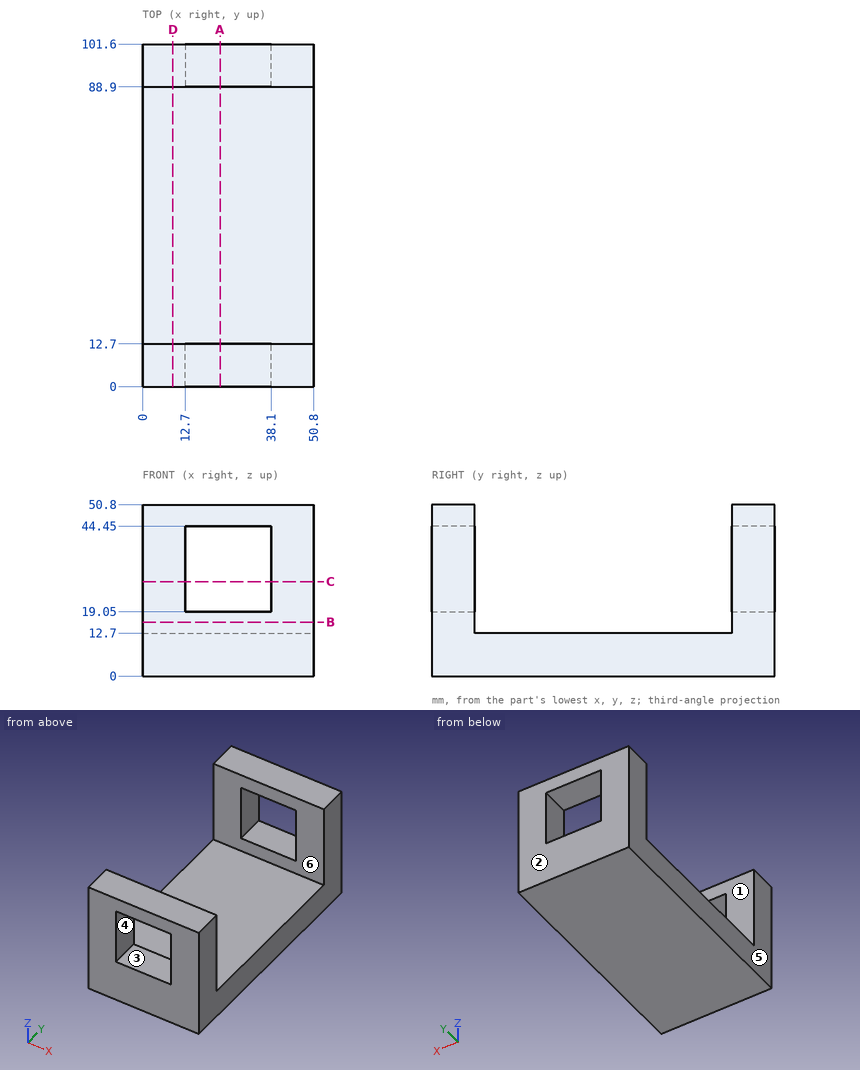
Design review of the part shown in the three views and the two pictorial views. Dimensions are in mm from the part's minimum x, y and z. A direction names the side the tool comes from. Give positions to 0.01 mm unless a question says otherwise; leave off trailing zeros. Loops run counter-clockwise (first coordinate to the right, second up) from the corner with the lowest first, then second, coordinate; pieces in that order, holes last. Notation, with made-up numbers: (-4.5, -3.5) -> (10.5, -3.5) arc R37 ccw to (10.5, 34.5) -> close; hole circle Ø3 at (54, 20). An arc over 180 degrees is marked (long way). Put each result on its own line as item: value. Start each with the question number.
1. Mouldability with a two-part tool opening along Y and no side actions: class the marked faces 1, 2 and 3 as released by +Y, released by -Y, zero draft, split by the parting line, or undercut.
2. For the marked faces 4, 5 and 6, list the 3-axis set-ups (+Z, -Z, +X, -X, +Y, -Y) from which the entire face can be reached by the end or side of a thin tool; tool diameter is ignored.
3. Clearance check with a flat-ended pin moving along its axis: P1, Ø15, axis at x = 38, y = 49, coming from the +Z side. State where the tip first meets the part, or that it passes through.
4. We need section B-B on z = 16. State the section outline as (x, y) points, then the cut area to 3 significant figures.
5. Wall thickness on probe 1 along Y at (x, z) = (34, 48); probe 2 along X at (y, z) = (11, 24.5); probe 3 along Z at (x, y) = (33.5, 4.5): over which ranges is each line inside the solid? List them lowest first.
6. We need section A-A on x = 23. State the section outline as (y, z) points.
7. We need section D-D on x = 9. State the section outline as (y, z) points.
8. We need section C-C on z = 28. State the section outline as (x, y) points, then the cut area to 3 significant figures.
Determined:
1. face 1: undercut
1. face 2: released by +Y
1. face 3: zero draft
2. face 4: +Y, -Y
2. face 5: +Z, -Z, -X, +Y, -Y
2. face 6: +Z, +X, -X
3. P1: z = 12.7
4. outline: (0, 0) -> (50.8, 0) -> (50.8, 12.7) -> (0, 12.7) -> close; (0, 88.9) -> (50.8, 88.9) -> (50.8, 101.6) -> (0, 101.6) -> close
4. area: 1,290 mm^2
5. probe 1: 0 to 12.7, 88.9 to 101.6
5. probe 2: 0 to 12.7, 38.1 to 50.8
5. probe 3: 0 to 19.05, 44.45 to 50.8
6. outline: (0, 0) -> (101.6, 0) -> (101.6, 19.05) -> (88.9, 19.05) -> (88.9, 12.7) -> (12.7, 12.7) -> (12.7, 19.05) -> (0, 19.05) -> close; (0, 44.45) -> (12.7, 44.45) -> (12.7, 50.8) -> (0, 50.8) -> close; (88.9, 44.45) -> (101.6, 44.45) -> (101.6, 50.8) -> (88.9, 50.8) -> close
7. outline: (0, 0) -> (101.6, 0) -> (101.6, 50.8) -> (88.9, 50.8) -> (88.9, 12.7) -> (12.7, 12.7) -> (12.7, 50.8) -> (0, 50.8) -> close
8. outline: (0, 0) -> (12.7, 0) -> (12.7, 12.7) -> (0, 12.7) -> close; (0, 88.9) -> (12.7, 88.9) -> (12.7, 101.6) -> (0, 101.6) -> close; (38.1, 0) -> (50.8, 0) -> (50.8, 12.7) -> (38.1, 12.7) -> close; (38.1, 88.9) -> (50.8, 88.9) -> (50.8, 101.6) -> (38.1, 101.6) -> close
8. area: 645 mm^2
